Design review of the part built by this model. Coordinates are the model's own, in mm. Face numbers are marked on the shaded views. A direction names the side the tool comes from. Coordinates: 2 decimals unless noted, no trailing zeros. Write each loop counter-clockwise with the first axis right and the second up, starting at its lowest first coordinate (ties: lowest second). Pieces come first, ordered by that corner, then holes. Notation, with made-up numbers: (84, 47.25) -> (131, 47.25) arc R13 ccw to (131, 71.25) -> close; hole circle Ø1 at (76, 22). An arc over 180 degrees is marked (long way). One line per question, with ' | ' between items. Start each with the question number.
Q1. Draft analysis for pull direction Z (two halves, no side actions). For the marked faces 1, 2, 3 and 4, state which applies: pulls with the +Z half, pulls with the -Z half, needs draft (parallel to the pull), parting line crosses it, or undercut.
Q2. Wall thickness on probe 1 along X at (y, z) = (-36, 14); probe 2 along X at (y, z) = (-34.5, 16); probe 3 along Z at (x, y) = (0, 0.75): over which ranges is each line inside the solid? List them lowest first.
Q3. Add section C-C on x = 23.5. State the section outline as (y, z) points.
Q4. For P1, Ø13.5, axis at x = 0, z = 0, coming from the +Y side; P2, Ø1, axis at y = -33.5, z = 15, coming from the -X side; P3, Ø4, axis at y = -51.5, z = -19, coming from the -X side; P4, Ø13.5, axis at x = -2, z = -0.5, coming from the +Y side, all flat-tipped, find the tip position at first contact; note any pin that passes through.
Q5. Add section D-D on z = -12.5. State the section outline as (x, y) points, and give its area (3 significant figures).
Q6. For the marked faces 5, 6 and 7, list the 3-axis set-ups (+Z, -Z, +X, -X, +Y, -Y) from which the entire face can be reached by the end or side of a thin tool; tool diameter is ignored.
from build123d import *

# Parameters (mm, degrees)
F0_R     = 30
F0_R_2   = 8.5
F1_DEPTH = 2.5
F3_DEPTH = 60
F4_DEPTH = 40


with BuildPart() as f1:
    # F0 (on Front) → F1 (new body)
    with BuildSketch(Plane.XZ):
        Circle(F0_R)
        Circle(F0_R_2, mode=Mode.SUBTRACT)
    extrude(amount=-F1_DEPTH)

    # F2 (on Front) → F3 (join)
    with BuildSketch(Plane.XZ):
        with BuildLine():
            ThreePointArc((9.9539621754, -0.9584555339), (9.9884839128, -0.4797802861), (10, 0))
            ThreePointArc((10, 0), (9.9474412154, 1.0239205366), (9.790317347, 2.0370778693))
            ThreePointArc((9.790317347, 2.0370778693), (9.0162927853, 4.3250970404), (7.7162445614, 6.3607837464))
            ThreePointArc((7.7162445614, 6.3607837464), (6.6748253827, 7.4462545021), (5.4823682108, 8.3632313612))
            ThreePointArc((5.4823682108, 8.3632313612), (3.3171763231, 9.4337872163), (0.9584555339, 9.9539621754))
            ThreePointArc((0.9584555339, 9.9539621754), (-0.5454827615, 9.9851113442), (-2.0370778693, 9.790317347))
            ThreePointArc((-2.0370778693, 9.790317347), (-4.3250970404, 9.0162927853), (-6.3607837464, 7.7162445614))
            ThreePointArc((-6.3607837464, 7.7162445614), (-7.4462545021, 6.6748253827), (-8.3632313612, 5.4823682108))
            ThreePointArc((-8.3632313612, 5.4823682108), (-9.4337872163, 3.3171763231), (-9.9539621754, 0.9584555339))
            ThreePointArc((-9.9539621754, 0.9584555339), (-9.9851113442, -0.5454827615), (-9.790317347, -2.0370778693))
            ThreePointArc((-9.790317347, -2.0370778693), (-9.0162927853, -4.3250970404), (-7.7162445614, -6.3607837464))
            ThreePointArc((-7.7162445614, -6.3607837464), (-6.6748253827, -7.4462545021), (-5.4823682108, -8.3632313612))
            ThreePointArc((-5.4823682108, -8.3632313612), (-3.3171763231, -9.4337872163), (-0.9584555339, -9.9539621754))
            ThreePointArc((-0.9584555339, -9.9539621754), (0.5454827615, -9.9851113442), (2.0370778693, -9.790317347))
            ThreePointArc((2.0370778693, -9.790317347), (4.3250970404, -9.0162927853), (6.3607837464, -7.7162445614))
            ThreePointArc((6.3607837464, -7.7162445614), (7.4462545021, -6.6748253827), (8.3632313612, -5.4823682108))
            ThreePointArc((8.3632313612, -5.4823682108), (9.4337872163, -3.3171763231), (9.9539621754, -0.9584555339))
        make_face()
        with BuildLine():
            ThreePointArc((-8.3632313612, 5.4823682108), (-7.4462545021, 6.6748253827), (-6.3607837464, 7.7162445614))
            Line((-6.3607837464, 7.7162445614), (-18.7140811189, 18.0494644761))
            ThreePointArc((-18.7140811189, 18.0494644761), (-19.7242264231, 16.9397429736), (-20.6686668466, 15.7735921965))
            Line((-20.6686668466, 15.7735921965), (-8.3632313612, 5.4823682108))
        make_face()
        with BuildLine():
            Line((-15.7735921965, -20.6686668466), (-5.4823682108, -8.3632313612))
            ThreePointArc((-5.4823682108, -8.3632313612), (-6.6748253827, -7.4462545021), (-7.7162445614, -6.3607837464))
            Line((-7.7162445614, -6.3607837464), (-18.0494644761, -18.7140811189))
            ThreePointArc((-18.0494644761, -18.7140811189), (-16.9397429736, -19.7242264231), (-15.7735921965, -20.6686668466))
        make_face()
        with BuildLine():
            Line((3.4613404795, -25.7685684912), (2.0370778693, -9.790317347))
            ThreePointArc((2.0370778693, -9.790317347), (0.5454827615, -9.9851113442), (-0.9584555339, -9.9539621754))
            Line((-0.9584555339, -9.9539621754), (0.469954935, -25.9957523907))
            ThreePointArc((0.469954935, -25.9957523907), (1.9689271292, -25.9253413856), (3.4613404795, -25.7685684912))
        make_face()
        with BuildLine():
            Line((20.6686668466, -15.7735921965), (8.3632313612, -5.4823682108))
            ThreePointArc((8.3632313612, -5.4823682108), (7.4462545021, -6.6748253827), (6.3607837464, -7.7162445614))
            Line((6.3607837464, -7.7162445614), (18.7140811189, -18.0494644761))
            ThreePointArc((18.7140811189, -18.0494644761), (19.7242264231, -16.9397429736), (20.6686668466, -15.7735921965))
        make_face()
        with BuildLine():
            ThreePointArc((9.790317347, 2.0370778693), (9.9474412154, 1.0239205366), (10, 0))
            ThreePointArc((10, 0), (9.9884839128, -0.4797802861), (9.9539621754, -0.9584555339))
            Line((9.9539621754, -0.9584555339), (25.9957523907, 0.469954935))
            ThreePointArc((25.9957523907, 0.469954935), (25.9253413856, 1.9689271292), (25.7685684912, 3.4613404795))
            Line((25.7685684912, 3.4613404795), (9.790317347, 2.0370778693))
        make_face()
        with BuildLine():
            ThreePointArc((5.4823682108, 8.3632313612), (6.6748253827, 7.4462545021), (7.7162445614, 6.3607837464))
            Line((7.7162445614, 6.3607837464), (18.0494644761, 18.7140811189))
            ThreePointArc((18.0494644761, 18.7140811189), (16.9397429736, 19.7242264231), (15.7735921965, 20.6686668466))
            Line((15.7735921965, 20.6686668466), (5.4823682108, 8.3632313612))
        make_face()
        with BuildLine():
            ThreePointArc((-2.0370778693, 9.790317347), (-0.5454827615, 9.9851113442), (0.9584555339, 9.9539621754))
            Line((0.9584555339, 9.9539621754), (-0.469954935, 25.9957523907))
            ThreePointArc((-0.469954935, 25.9957523907), (-1.9689271292, 25.9253413856), (-3.4613404795, 25.7685684912))
            Line((-3.4613404795, 25.7685684912), (-2.0370778693, 9.790317347))
        make_face()
        with BuildLine():
            ThreePointArc((-9.790317347, -2.0370778693), (-9.9851113442, -0.5454827615), (-9.9539621754, 0.9584555339))
            Line((-9.9539621754, 0.9584555339), (-25.9957523907, -0.469954935))
            ThreePointArc((-25.9957523907, -0.469954935), (-25.9253413856, -1.9689271292), (-25.7685684912, -3.4613404795))
            Line((-25.7685684912, -3.4613404795), (-9.790317347, -2.0370778693))
        make_face()
    extrude(amount=F3_DEPTH)

    # F4 (cut): a face of the model
    f4_faces = [f1.faces().sort_by_distance(p)[0] for p in [
        (0, 0, 0),
    ]]
    extrude(f4_faces, amount=-F4_DEPTH, mode=Mode.SUBTRACT)


solid = f1.part
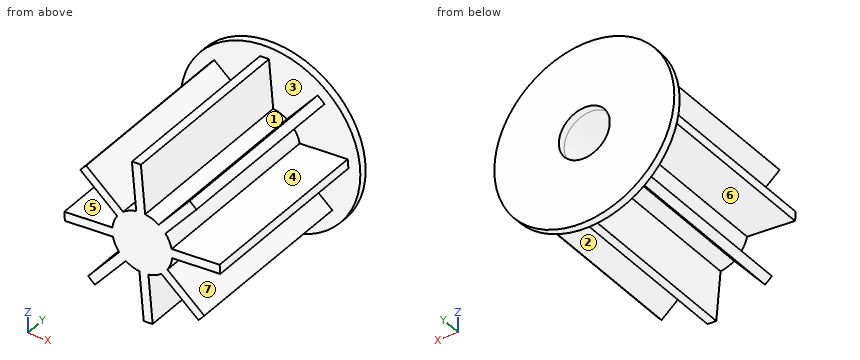
Output values:
1) face 1: pulls with the +Z half | face 2: pulls with the -Z half | face 3: undercut | face 4: undercut
2) probe 1: x = -18.55 to -13.87, -2.41 to 0.6, 10.2 to 14.11 | probe 2: x = -20.49 to -16.26, -2.59 to 0.42, 11.87 to 15.78 | probe 3: z = -30 to -8.5, 8.5 to 30
3) outline: (-60, 0.25) -> (0, 0.25) -> (0, -18.65) -> (2.5, -18.65) -> (2.5, 18.65) -> (0, 18.65) -> (0, 3.26) -> (-60, 3.26) -> close
4) P1: stops at y = -40 | P2: stops at x = -20.34 | P3: stops at x = -18.05 | P4: stops at y = 2.5
5) outline: (-27.27, 0) -> (-12.85, 0) -> (-12.85, -60) -> (-8.94, -60) -> (-8.94, 0) -> (-0.73, 0) -> (-0.73, -60) -> (2.28, -60) -> (2.28, 0) -> (12.08, 0) -> (12.08, -60) -> (16.75, -60) -> (16.75, 0) -> (27.27, 0) -> (27.27, 2.5) -> (-27.27, 2.5) -> close | area: 832 mm2
6) face 5: -X, -Y | face 6: -Y | face 7: +X, -Y
